```python
from build123d import *

# Parameters (mm, degrees)
SKETCH1_R           = 10
BOSS_EXTRUDE1_DEPTH = 10
SKETCH2_W           = 30.028941415
SKETCH2_H           = 40
BOSS_EXTRUDE2_DEPTH = 20
SKETCH3_OUTSIDE_W   = 59.204
SKETCH3_OUTSIDE_H   = 49.204
CUT_EXTRUDE1_DEPTH  = 36
CUT_EXTRUDE2_DEPTH  = 20


with BuildPart() as part:
    # Sketch1 → Boss-Extrude1 (new body)
    with BuildSketch(Plane(origin=(0, 0, 0), x_dir=(1, 0, 0), z_dir=(0, 1, 0))):
        with BuildLine():
            Line((0, 20), (-50, 20))
            Line((-50, 20), (-50, -20))
            Line((-50, -20), (0, -20))
            ThreePointArc((0, -20), (20, 0), (0, 20))
        make_face()
        with Locations(Location((0, 0, 0), (0, 0, 270))):
            Circle(SKETCH1_R, mode=Mode.SUBTRACT)
    extrude(amount=BOSS_EXTRUDE1_DEPTH)

    # Sketch2 → Boss-Extrude2 (add)
    with BuildSketch(Plane(origin=(0, 10, 0), x_dir=(1, 0, 0), z_dir=(0, 1, 0))):
        with Locations((-34.985529293, 0)):
            Rectangle(SKETCH2_W, SKETCH2_H)
    extrude(amount=BOSS_EXTRUDE2_DEPTH)

    # Sketch3 outside → Cut-Extrude1 (cut)
    with BuildSketch(Plane(origin=(-19.971058585, 0, 0), x_dir=(0, 0, -1), z_dir=(1, 0, 0))):
        with Locations((0, 15)):
            Rectangle(SKETCH3_OUTSIDE_W, SKETCH3_OUTSIDE_H)
        Polygon((20, 30), (10, 30), (-20, 20), (-20, 0), (20, 0), align=None, mode=Mode.SUBTRACT)
    extrude(amount=-CUT_EXTRUDE1_DEPTH, mode=Mode.SUBTRACT)

    # Sketch4 → Cut-Extrude2 (cut)
    with BuildSketch(Plane(origin=(0, 30, 0), x_dir=(1, 0, 0), z_dir=(0, 1, 0))):
        Polygon((-19.971058585, -20), (-19.971058585, 10), (-39.971058585, -20), align=None)
    extrude(amount=-CUT_EXTRUDE2_DEPTH, mode=Mode.SUBTRACT)


solid = part.part
```
Build history of the part. All positions in model axes, mm. A direction names the side the tool comes from. Give positions to 0.01 mm unless a question says otherwise; leave off trailing zeros. Order: outer loops, then holes, each group sorted by start corner. A loop starts at its lowest first (then second) coordinate and runs counter-clockwise, first axis right, second up. Notation, with made-up numbers: M 87.25,19 L 96.25,19 A30 ccw 96.25,42 Z; hole C 85.5,-15 d2. An arc over 180 degrees is marked long. Write item = value, one per line. Start each with the question number.
(1) Two-plate mould, pull along Z, no slides. Class faces 1 (the cylindrical face through (-9.76, 4.93, -2.17)), 2 (the flat face through (-38.11, 26.18, 1.46)), 3 (the flat face through (-19.971, 20, -15)): released by +Z, released by -Z, zero draft, split by the parting line, or undercut.
(2) Slice it at C-C on y = 13.25. Write the cut outline in (x, z).
(3) Slice it at A-A on z = 2. Write the cut outline in (x, y), plus the area to 4 significant figures.
(4) Slice it at D-D on x = -43. Write the cut outline in (y, z), plus the area to 3 significant figures.
(5) Pin check, flat tips, straight feed: pin 1 Ø11 at (y, z) = (23, -17) entering from +X; pin 2 Ø12 at (x, z) = (-23, -0.5) entering from +Y; pin 3 Ø5 at (x, z) = (-10, 15.5) entering from +Y; pin 4 Ø3 at (x, z) = (-25.5, -2.5) entering from -Y. Stop position of each tip, or through.
(6) Which spindle directions (+Z, -Z, +X, -X, +Y, -Y) get a long thin tool onto all of the face, cutting with end or side? Do faces 4 (the flat face through (-29.83, 17.92, 4.79)), 5 (the flat face through (-31, 8, 20)). Say none if no direction does.
(7) Slice it at B-B on y = 2.5. Write the cut outline in (x, z).
(8) Probe L1, parallel to X at y = 11.25, z = -17; L2, parallel to X at y = 6.5, z = 0; L3, parallel to Y at x = 14.5, z = 5. List the from-to ranges inside material, lowest first. Write a range as [from, to].
Responses:
q1.face_1 = undercut
q1.face_2 = released by +Z
q1.face_3 = zero draft
q2.outline = M -50,-20 L -19.97,-20 L -19.97,-10 L -39.97,20 L -50,20 Z
q3.outline = M -50,0 L -9.8,0 L -9.8,10 L -27.97,10 L -27.97,26 L -50,26 Z; M 9.8,0 L 19.9,0 L 19.9,10 L 9.8,10 Z
q3.area = 855.5 mm2
q4.outline = M 0,-20 L 30,-20 L 30,-10 L 20,20 L 0,20 Z
q4.area = 1,050 mm2
q5.pin_1 = -19.97
q5.pin_2 = 28.83
q5.pin_3 = 10
q5.pin_4 = 0
q6.face_4 = +Z, +X, +Y
q6.face_5 = +Z, +X, -X, +Y, -Y
q7.outline = M -50,-20 L 0,-20 A20 ccw 0,20 L -50,20 Z; hole C 0,0 d20
q8.L1 = [-50, -19.97]
q8.L2 = [-50, -10], [10, 20]
q8.L3 = [0, 10]
